Autodesk Inventor part; units mm, degrees
ref_plane "YZ Plane" through (0, 0, 0) normal (1, 0, 0) x (0, 1, 0)
ref_plane "XZ Plane" through (0, 0, 0) normal (0, 1, 0) x (-1, 0, 0)
ref_plane "XY Plane" through (0, 0, 0) normal (0, 0, 1) x (1, 0, 0)
sketch "スケッチ1" plane through (0, 0, 0) normal (0, 0, 1) x (1, 0, 0)
  circle A0 centre (0, 0) radius 13.75
  dimension "d0" = 27.5
extrude "押し出し1" add sketch "スケッチ1" along normal blind 38
sketch "スケッチ2" plane through (0, 0, 38) normal (0, 0, 1) x (1, 0, 0)
  circle A0 centre (0, 0) radius 15
  dimension "d3" = 30
extrude "押し出し2" add sketch "スケッチ2" along normal blind 2
sketch "スケッチ3" plane through (0, 0, 40) normal (0, 0, 1) x (1, 0, 0)
  circle A0 centre (0, 0) radius 18.5
  dimension "d6" = 37
extrude "押し出し3" add sketch "スケッチ3" along normal blind 27.5
sketch "スケッチ4" plane through (0, 0, 0) normal (0, 0, -1) x (-1, 0, 0)
  circle A0 centre (0, 0) radius 5.1
  dimension "d9" = 10.2
extrude "押し出し4" add sketch "スケッチ4" along normal blind 3
sketch "スケッチ5" plane through (0, 0, 67.5) normal (0, 0, 1) x (1, 0, 0)
  circle A0 centre (-7, 0) radius 6
  point P0 (0, 0)
  dimension "d12" = 12
extrude "押し出し5" add sketch "スケッチ5" along normal blind 6
sketch "スケッチ6" plane through (-7, 0, 73.5) normal (0, 0, 1) x (1, 0, 0)
  circle A0 centre (0, 0) radius 3
  point P0 (7, 0)
  dimension "d15" = 6
extrude "押し出し6" add sketch "スケッチ6" along normal blind 15
sketch "スケッチ7" plane through (0, 0, 67.5) normal (0, 0, 1) x (1, 0, 0)
  circle A0 centre (-7.75, -13.4234) radius 1.5
  circle A1 centre (-7.75, 13.4234) radius 1.5
  circle A2 centre (15.5, 0) radius 1.5
  circle A3 centre (0, -15.5) radius 1.5
  circle A4 centre (-13.4234, 7.75) radius 1.5
  circle A5 centre (13.4234, 7.75) radius 1.5
  point P0 (0, 0)
  point P1 (0, 0)
  point P2 (0, 0)
  dimension "d19" = 3
  dimension "d20" = 3
  dimension "d21" = 3
  dimension "d22" = 3
  dimension "d23" = 3
  dimension "d24" = 3
extrude "押し出し7" cut sketch "スケッチ7" against normal blind 15 contours A3 | A4 | A5
sketch "スケッチ8" plane through (0, 0, 67.5) normal (0, 0, 1) x (1, 0, 0)
  circle A0 centre (-7.75, -13.4234) radius 1.5
  circle A1 centre (-7.75, 13.4234) radius 1.5
  circle A2 centre (15.5, 0) radius 1.5
  circle A3 centre (0, -15.5) radius 1.5
  circle A4 centre (-13.4234, 7.75) radius 1.5
  circle A5 centre (13.4234, 7.75) radius 1.5
  point P0 (0, 0)
  point P1 (0, 0)
  point P2 (0, 0)
  point P3 (0, 0)
  dimension "d27" = 3
  dimension "d28" = 3
  dimension "d29" = 3
  dimension "d30" = 3
  dimension "d31" = 3
  dimension "d32" = 3
extrude "押し出し8" cut sketch "スケッチ8" against normal blind 1 contours A0 | A1 | A2
properties part number "380-300c1" material "ステンレス鋼"
The model under review builds one solid part; all positions refer to its coordinate system, in mm. A direction names the side the tool comes from. Round coordinates to 2 decimals unless told otherwise and drop trailing zeros. Loops run counter-clockwise (first coordinate to the right, second up) from the corner with the lowest first, then second, coordinate; pieces in that order, holes last.
1) Consider section A-A on y = 0. State the section outline as (x, z) points.
Values follow:
outline: (-18.5, 40) - (-15, 40) - (-15, 38) - (-13.75, 38) - (-13.75, 0) - (-5.1, 0) - (-5.1, -3) - (5.1, -3) - (5.1, 0) - (13.75, 0) - (13.75, 38) - (15, 38) - (15, 40) - (18.5, 40) - (18.5, 67.5) - (17, 67.5) - (17, 66.5) - (14, 66.5) - (14, 67.5) - (-1, 67.5) - (-1, 73.5) - (-4, 73.5) - (-4, 88.5) - (-10, 88.5) - (-10, 73.5) - (-13, 73.5) - (-13, 67.5) - (-18.5, 67.5) - close
2) Tool access review of faces 4 (the face through (0, -6, 0)), 5 (the face through (-14.614, 6.837, 60.105)): name each direction out of +Z, -Z, +X, -X, +Y, -Y from which nothing blocks a thin tool from reaching the whole face with its end or side.
Values follow:
face 4: -Z
face 5: +Z
3) The part is to be moulded in two halves that separate along X. For faces 1 (the face through (-4.01, 18.06, 53.56)), 2 (the face through (-8, 13, 66.5)), 3 (the face through (-10, -1, 73.5)), say which applies: pulls with the +X half, pulls with the -X half, needs draft (parallel to the pull), parting line crosses it, or undercut.
Values follow:
face 1: parting line crosses it
face 2: undercut
face 3: needs draft
4) Consider section D-D on x = -7.75. State the section outline as (y, z) points, then the cut area to 3 significant figures.
Values follow:
outline: (-16.8, 40) - (-12.84, 40) - (-12.84, 38) - (-11.36, 38) - (-11.36, 0) - (11.36, 0) - (11.36, 38) - (12.84, 38) - (12.84, 40) - (16.8, 40) - (16.8, 67.5) - (14.92, 67.5) - (14.92, 66.5) - (11.92, 66.5) - (11.92, 67.5) - (5.95, 67.5) - (5.95, 73.5) - (2.9, 73.5) - (2.9, 88.5) - (-2.9, 88.5) - (-2.9, 73.5) - (-5.95, 73.5) - (-5.95, 67.5) - (-11.92, 67.5) - (-11.92, 66.5) - (-14.92, 66.5) - (-14.92, 67.5) - (-16.8, 67.5) - close
area: 1,990 mm2
5) Consider section C-C on z = 41.5. State the section outline as (x, y) points.
Values follow:
outline: circle Ø37 at (0, 0)
6) Consider section B-B on x = 0.5. State the section outline as (y, z) points.
Values follow:
outline: (-18.49, 40) - (-14.99, 40) - (-14.99, 38) - (-13.74, 38) - (-13.74, 0) - (-5.08, 0) - (-5.08, -3) - (5.08, -3) - (5.08, 0) - (13.74, 0) - (13.74, 38) - (14.99, 38) - (14.99, 40) - (18.49, 40) - (18.49, 67.5) - (-14.09, 67.5) - (-14.09, 52.5) - (-16.91, 52.5) - (-16.91, 67.5) - (-18.49, 67.5) - close
7) Wall thickness on line 1 along X through (y, z) = (8, 67); line 2 along X through (y, z) = (7, 61); line 3 along Z through (x, y) = (2.5, 11.5): over which ranges is each line inside the solid? List them lowest first.
Values follow:
line 1: x = -16.68 to -14.9, -11.94 to 11.94, 14.9 to 16.68
line 2: x = -17.12 to -14.72, -12.12 to 12.12, 14.72 to 17.12
line 3: z = 0 to 67.5
8) Clearance check with flat-ended pins moving along their axes: P1, Ø1.5, axis at x = -8, y = -13, coming from the +Z side; P2, Ø2, axis at x = -11.5, z = 63, coming from the -Y side; P3, Ø10, axis at x = 10.5, y = -14, coming from the -Z side. State where each tip first meets the part, or that it passes through.
Values follow:
P1: stops at z = 66.5
P2: stops at y = -15.23
P3: stops at z = 0
